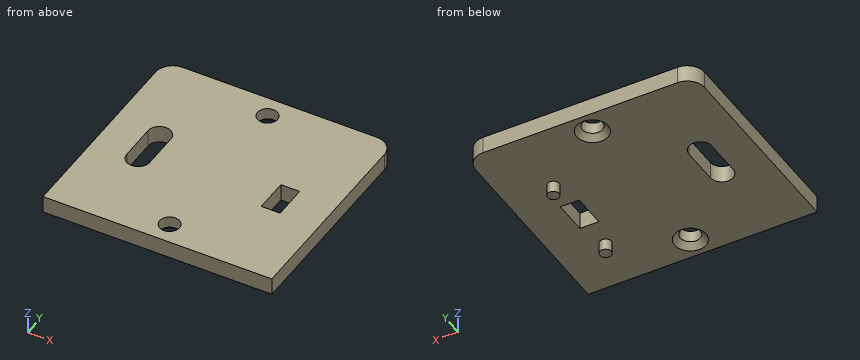
```python
from build123d import *

# Parameters (mm, degrees)
ESQUISSE1_W             = 40
ESQUISSE1_H             = 37.5
ESQUISSE1_R             = 1.75
BOSS_EXTRU_1_DEPTH      = 3
CHANFREIN1_SIZE         = 1
CONG_1_R                = 3
ESQUISSE5_W             = 3.3
ESQUISSE5_H             = 6
ENL_V_MAT_EXTRU_2_DEPTH = 42.208509496
ESQUISSE6_R             = 1
BOSS_EXTRU_2_DEPTH      = 2


with BuildPart() as part:
    # Esquisse1 → Boss.-Extru.1 (new body)
    with BuildSketch(Plane.XY):
        with Locations((-10.738255034, 8.531879195)):
            Rectangle(ESQUISSE1_W, ESQUISSE1_H)
        with Locations((-10.738255034, -6.468120805)):
            Circle(ESQUISSE1_R, mode=Mode.SUBTRACT)
        with Locations((-10.738255034, 23.531879195)):
            Circle(ESQUISSE1_R, mode=Mode.SUBTRACT)
    extrude(amount=BOSS_EXTRU_1_DEPTH)

    # Chanfrein1
    chanfrein1_edges = [part.edges().sort_by_distance(p)[0] for p in [
        (-12.488255034, -6.468120805, 0),
        (-12.488255034, 23.531879195, 0),
    ]]
    chamfer(chanfrein1_edges, length=CHANFREIN1_SIZE)

    # Congé1
    cong_1_edges = [part.edges().sort_by_distance(p)[0] for p in [
        (-30.738255034, 27.281879195, 1.5),
        (9.261744966, 27.281879195, 1.5),
    ]]
    fillet(cong_1_edges, radius=CONG_1_R)

    # Esquisse5 → Enlèv. mat.-Extru.2 (cut, through all)
    with BuildSketch(Plane(origin=(0, 0, 0), x_dir=(-1, 0, 0), z_dir=(0, 0, -1))):
        with BuildLine():
            Line((24.738255034, 11.451981866), (24.738255034, 4.951981866))
            ThreePointArc((24.738255034, 4.951981866), (22.738255034, 2.951981866), (20.738255034, 4.951981866))
            Line((20.738255034, 4.951981866), (20.738255034, 11.451981866))
            ThreePointArc((20.738255034, 11.451981866), (22.738255034, 13.451981866), (24.738255034, 11.451981866))
        make_face()
        with Locations((-0.860681094, 7.158115812)):
            Rectangle(ESQUISSE5_W, ESQUISSE5_H)
    extrude(amount=-ENL_V_MAT_EXTRU_2_DEPTH, mode=Mode.SUBTRACT)

    # Esquisse6 → Boss.-Extru.2 (add)
    with BuildSketch(Plane(origin=(0, 0, 0), x_dir=(-1, 0, 0), z_dir=(0, 0, -1))):
        with Locations(Location((-0.860681094, 15.158115812, 0), (0, 0, 180))):
            Circle(ESQUISSE6_R)
        with Locations(Location((-0.860681094, -0.841884188, 0), (0, 0, 180))):
            Circle(ESQUISSE6_R)
    extrude(amount=BOSS_EXTRU_2_DEPTH)


solid = part.part
```
Can you work these out from the model? Positions are in its coordinate system, mm. Coordinates: 2 decimals unless noted, no trailing zeros. Loops run counter-clockwise (first coordinate to the right, second up) from the corner with the lowest first, then second, coordinate; pieces in that order, holes last.
Item 1: I'm going to push flat-ended pins straight in: pin 1 (3 mm diameter, centred on x = -19, y = 1, fed in from -Z); pin 2 (4 mm diameter, centred on x = -10.74, y = -6.47, fed in from -Z). Where does each tip first touch, or does it pass through?
Answers below:
pin 1: stops at z = 0
pin 2: stops at z = 0.75
Item 2: Suppose I cut it at A-A (y = 8). Please give me the cut outline in (x, z).
Answers below:
outline: (-30.74, 0) - (-24.74, 0) - (-24.74, 3) - (-30.74, 3) - close; (-20.74, 0) - (-0.79, 0) - (-0.79, 3) - (-20.74, 3) - close; (2.51, 0) - (9.26, 0) - (9.26, 3) - (2.51, 3) - close
Item 3: Suppose I cut it at C-C (x = -7). Please give me the cut outline in (y, z), then the cut area to 4 significant figures.
Answers below:
outline: (-10.22, 0) - (27.28, 0) - (27.28, 3) - (-10.22, 3) - close
area: 112.5 mm2
Item 4: Please list where these lines run through material, in increasing order: L1, parallel to X at y = 11, z = 1.75; L2, parallel to Z at x = -14.5, y = 20; L3, parallel to X at y = -8, z = 0.3.
Answers below:
L1: x = -30.74 to -24.74, -20.74 to 9.26
L2: z = 0 to 3
L3: x = -30.74 to -12.65, -8.83 to 9.26
Item 5: Suppose I cut it at D-D (z = -1.55). Please give me the cut outline in (x, y).
Answers below:
outline: circle Ø2 at (0.86, -0.84); circle Ø2 at (0.86, 15.16)
Item 6: Suppose I cut it at B-B (z = 1.65). Please give me the cut outline in (x, y).
Answers below:
outline: (-30.74, -10.22) - (9.26, -10.22) - (9.26, 24.28) arc R3 ccw to (6.26, 27.28) - (-27.74, 27.28) arc R3 ccw to (-30.74, 24.28) - close; hole (-24.74, 4.95) arc R2 ccw to (-20.74, 4.95) - (-20.74, 11.45) arc R2 ccw to (-24.74, 11.45) - close; hole circle Ø3.5 at (-10.74, -6.47); hole circle Ø3.5 at (-10.74, 23.53); hole (-0.79, 4.16) - (2.51, 4.16) - (2.51, 10.16) - (-0.79, 10.16) - close
